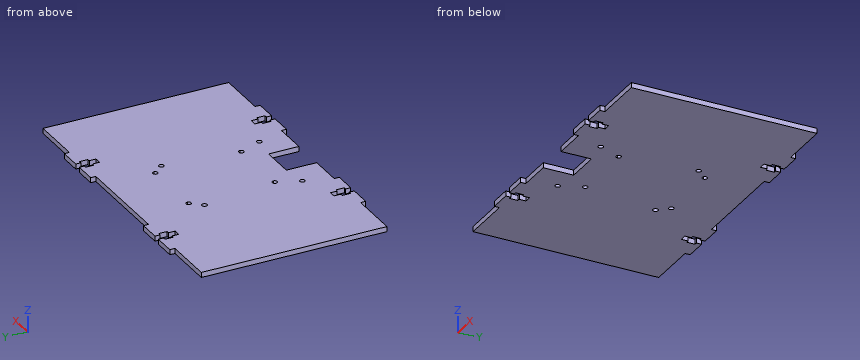
from build123d import *

# Parameters (mm, degrees)
SKETCH_1_W          = 28
SKETCH_1_H          = 42.5
SKETCH_1_R          = 1.5
EXTRUDE_1_DEPTH     = 3
SKETCH1_W           = 20.227510382
SKETCH1_H           = 18
CUT_EXTRUDE1_DEPTH  = 10
CUT_EXTRUDE_1_DEPTH = 213.55117031


with BuildPart() as part:
    # 草图1 → 凸台-拉伸1 (new body)
    # profile 1 of 16: a face of its own
    with BuildSketch(Plane.XY):
        Polygon((41.5, 0), (43, 0), (43, 3), (30, 3), (30, 0), align=None)
    # profile 2 of 16: a face of its own
    with BuildSketch(Plane.XY):
        Polygon((48.5, 0), (60, 0), (60, 3), (47, 3), (47, 0), align=None)
    # profile 3 of 16: a face of its own
    with BuildSketch(Plane.XY):
        Polygon((120, 3), (120, 0), (131.5, 0), (133, 0), (133, 3), align=None)
    # profile 4 of 16: a face of its own
    with BuildSketch(Plane.XY):
        Polygon((137, 3), (137, 0), (138.5, 0), (150, 0), (150, 3), align=None)
    # profile 5 of 16: a face of its own
    with BuildSketch(Plane.XY):
        Polygon((120, 0), (90, 0), (90, -12.5), (118, -12.5), (118, -55), (180, -55), (180, 0), (150, 0), (138.5, 0), (138.5, -5), (137, -5), (137, -9), (133, -9), (133, -5), (131.5, -5), (131.5, 0), align=None)
    # profile 6 of 16: a face of its own
    with BuildSketch(Plane.XY):
        Polygon((90, -12.5), (90, 0), (60, 0), (48.5, 0), (48.5, -5), (47, -5), (47, -9), (43, -9), (43, -5), (41.5, -5), (41.5, 0), (30, 0), (0, 0), (0, -55), (62, -55), (62, -12.5), align=None)
    # profile 7 of 16: a face of its own
    with BuildSketch(Plane.XY):
        with Locations((76, -33.75)):
            Rectangle(SKETCH_1_W, SKETCH_1_H)
        with Locations((65.5, -36)):
            Circle(SKETCH_1_R, mode=Mode.SUBTRACT)
    # profile 8 of 16: a face of its own
    with BuildSketch(Plane.XY):
        with Locations((104, -33.75)):
            Rectangle(SKETCH_1_W, SKETCH_1_H)
        with Locations((114.5, -36)):
            Circle(SKETCH_1_R, mode=Mode.SUBTRACT)
    # profile 9 of 16: a face of its own
    with BuildSketch(Plane.XY):
        Polygon((41.5, -110), (30, -110), (30, -113), (43, -113), (43, -110), align=None)
    # profile 10 of 16: a face of its own
    with BuildSketch(Plane.XY):
        Polygon((60, -113), (60, -110), (48.5, -110), (47, -110), (47, -113), align=None)
    # profile 11 of 16: a face of its own
    with BuildSketch(Plane.XY):
        Polygon((131.5, -110), (120, -110), (120, -113), (133, -113), (133, -110), align=None)
    # profile 12 of 16: a face of its own
    with BuildSketch(Plane.XY):
        Polygon((150, -113), (150, -110), (138.5, -110), (137, -110), (137, -113), align=None)
    # profile 13 of 16: a face of its own
    with BuildSketch(Plane.XY):
        Polygon((118, -97.5), (90, -97.5), (90, -110), (120, -110), (131.5, -110), (131.5, -105), (133, -105), (133, -101), (137, -101), (137, -105), (138.5, -105), (138.5, -110), (150, -110), (180, -110), (180, -55), (118, -55), align=None)
    # profile 14 of 16: a face of its own
    with BuildSketch(Plane.XY):
        Polygon((90, -110), (90, -97.5), (62, -97.5), (62, -55), (0, -55), (0, -110), (30, -110), (41.5, -110), (41.5, -105), (43, -105), (43, -101), (47, -101), (47, -105), (48.5, -105), (48.5, -110), (60, -110), align=None)
    # profile 15 of 16: a face of its own
    with BuildSketch(Plane.XY):
        with Locations((76, -76.25)):
            Rectangle(SKETCH_1_W, SKETCH_1_H)
        with Locations((65.5, -94)):
            Circle(SKETCH_1_R, mode=Mode.SUBTRACT)
    # profile 16 of 16: a face of its own
    with BuildSketch(Plane.XY):
        with Locations((104, -76.25)):
            Rectangle(SKETCH_1_W, SKETCH_1_H)
        with Locations((114.5, -94)):
            Circle(SKETCH_1_R, mode=Mode.SUBTRACT)
    extrude(amount=EXTRUDE_1_DEPTH)

    # Sketch1 → Cut-Extrude1 (cut)
    with BuildSketch(Plane.XY.offset(3)):
        with Locations((90, -101)):
            Rectangle(SKETCH1_W, SKETCH1_H)
    extrude(amount=-CUT_EXTRUDE1_DEPTH, mode=Mode.SUBTRACT)

    # 草图2 → 切除-拉伸1 (cut, through all)
    with BuildSketch(Plane.XY.offset(3)):
        with BuildLine():
            ThreePointArc((72.5, -29.5), (69.939339828, -28.439339828), (71, -31))
            Line((71, -31), (71, -29.5))
            Line((71, -29.5), (72.5, -29.5))
        make_face()
        with BuildLine():
            Line((71, -29.5), (71, -31))
            ThreePointArc((71, -31), (72.060660172, -30.560660172), (72.5, -29.5))
            Line((72.5, -29.5), (71, -29.5))
        make_face()
        with BuildLine():
            ThreePointArc((107.5, -29.5), (107.939339828, -30.560660172), (109, -31))
            Line((109, -31), (109, -29.5))
            Line((109, -29.5), (107.5, -29.5))
        make_face()
        with BuildLine():
            Line((109, -29.5), (109, -31))
            ThreePointArc((109, -31), (110.060660172, -30.560660172), (110.5, -29.5))
            ThreePointArc((110.5, -29.5), (109, -28), (107.5, -29.5))
            Line((107.5, -29.5), (109, -29.5))
        make_face()
        with BuildLine():
            ThreePointArc((72.5, -80.5), (72.060660172, -79.439339828), (71, -79))
            Line((71, -79), (71, -80.5))
            Line((71, -80.5), (72.5, -80.5))
        make_face()
        with BuildLine():
            Line((71, -80.5), (71, -79))
            ThreePointArc((71, -79), (69.939339828, -81.560660172), (72.5, -80.5))
            Line((72.5, -80.5), (71, -80.5))
        make_face()
        with BuildLine():
            ThreePointArc((110.5, -80.5), (110.060660172, -79.439339828), (109, -79))
            Line((109, -79), (109, -80.5))
            Line((109, -80.5), (107.5, -80.5))
            ThreePointArc((107.5, -80.5), (109, -82), (110.5, -80.5))
        make_face()
        with BuildLine():
            Line((109, -80.5), (109, -79))
            ThreePointArc((109, -79), (107.939339828, -79.439339828), (107.5, -80.5))
            Line((107.5, -80.5), (109, -80.5))
        make_face()
    extrude(amount=-CUT_EXTRUDE_1_DEPTH, mode=Mode.SUBTRACT)


solid = part.part
Could you check a few things on this model? Use its own coordinates, in mm. Give positions to 0.01 mm unless a question says otherwise; leave off trailing zeros. Order: outer loops, then holes, each group sorted by start corner. A loop starts at its lowest first (then second) coordinate and runs counter-clockwise, first axis right, second up. Notation, with made-up numbers: (43.25, 40.5) - (97.25, 40.5) arc R23 cw to (97.25, 70.5) - close; hole circle Ø4 at (61, -2). An arc over 180 degrees is marked (long way). Return JSON: item names as keys, results as strings. Group by question number.
Q1. Suppose I cut it at B-B, the plane x = 162. Please give me the cut outline in (y, z).
Q2. Please list where these lines run through material, in increasing order: line 1 along Y through (x, z) = (65.5, 0.85); line 2 along X through (y, z) = (-80.5, 0.6); line 3 along Y through (x, z) = (71, 2.1). Write a range as [from, to].
Q3. Suppose I cut it at A-A, the plane z = 2.1. State how many separate pieces and enclosed holes the cut face has, and give its area (3 significant figures).
Q4. Will these pins go through, and if not, where does the flat tip stop? pin 1 Ø1.5 at (x, z) = (153.5, 2) entering from +Y; pin 2 Ø1.5 at (y, z) = (1.5, 1) entering from +X; pin 3 Ø3.5 at (x, y) = (65.5, -94) entering from +Z.
Resolved:
{
 "1": {"outline": "(-110, 0) - (0, 0) - (0, 3) - (-110, 3) - close"},
 "2": {"line 1": "y = [-110, -95.5], [-92.5, -37.5], [-34.5, 0]", "line 2": "x = [0, 69.5], [72.5, 107.5], [110.5, 180]", "line 3": "y = [-110, -82], [-79, -31], [-28, 0]"},
 "3": {"separate pieces": "1", "enclosed holes": "8", "area": "19,500 mm2"},
 "4": {"pin 1": "stops at y = 0", "pin 2": "stops at x = 150", "pin 3": "stops at z = 3"}
}
